Autodesk Inventor part; units mm, degrees
ref_plane "YZ Plane" through (0, 0, 0) normal (1, 0, 0) x (0, 1, 0)
ref_plane "XZ Plane" through (0, 0, 0) normal (0, 1, 0) x (-1, 0, 0)
ref_plane "XY Plane" through (0, 0, 0) normal (0, 0, 1) x (1, 0, 0)
sketch "スケッチ1" plane through (0, 0, 0) normal (0, 1, 0) x (-1, 0, 0)
  circle A0 centre (0, 0) radius 178.1675
  circle A1 centre (0, 0) radius 157.8276
  line L0 (168.1877, 0) -> (166.7488, -21.9529)
  line L1 (168.1877, 0) -> (130.1721, 2.4917) construction
  line L2 (249.4344, 0) -> (-249.4344, 0)
  line L3 (166.7488, -21.9529) -> (156.7702, -21.2989)
  line L4 (156.7702, -21.2989) -> (158.2091, 0.654) construction
  line L5 (158.2091, 0.654) -> (168.1877, 0)
  line L6 (157.4896, -10.3224) -> (0, 0)
  line L7 (166.7488, -21.9529) -> (162.4568, -43.5302)
  line L8 (162.4568, -43.5302) -> (152.649, -41.5793) construction
  line L9 (152.649, -41.5793) -> (156.9409, -20.002) construction
  line L10 (156.9409, -20.002) -> (166.7488, -21.9529) construction
  line L11 (162.4568, -43.5302) -> (155.3851, -64.3626)
  line L12 (155.3851, -64.3626) -> (145.9158, -61.1482) construction
  line L13 (145.9158, -61.1482) -> (152.9875, -40.3158) construction
  line L14 (152.9875, -40.3158) -> (162.4568, -43.5302) construction
  line L15 (155.3851, -64.3626) -> (145.6548, -84.0938)
  line L16 (145.6548, -84.0938) -> (136.6861, -79.6709) construction
  line L17 (136.6861, -79.6709) -> (146.4164, -59.9397) construction
  line L18 (146.4164, -59.9397) -> (155.3851, -64.3626) construction
  line L19 (0, 0) -> (111.6009, -111.6009)
  line L20 (145.6548, -84.0938) -> (137.3401, -78.5381) construction
  line L21 (137.3401, -78.5381) -> (125.1176, -96.8305) construction
  line L22 (125.1176, -96.8305) -> (133.4323, -102.3862) construction
  line L23 (133.4323, -102.3862) -> (145.6548, -84.0938)
  line L24 (133.4323, -102.3862) -> (125.9139, -95.7927) construction
  line L25 (125.9139, -95.7927) -> (111.4082, -112.3332) construction
  line L26 (111.4082, -112.3332) -> (118.9266, -118.9266)
  line L27 (118.9266, -118.9266) -> (133.4323, -102.3862)
  line L28 (111.6009, -111.6009) -> (118.9266, -118.9266)
  line L29 (166.7488, -21.9529) -> (176.7274, -22.6069) construction
  line L30 (118.9266, -118.9266) -> (125.9834, -125.9834)
  point P0 (154.795, -30.7906)
  point P1 (149.4517, -50.732)
  point P2 (141.5512, -69.8053)
  point P3 (131.2288, -87.6843)
  point P4 (118.661, -104.0629)
  point P5 (157.8276, 0)
  point P6 (178.1675, 0)
  dimension "d0" = 22
  dimension "d1" = 10
  dimension "d2" = 45
  dimension "d4" = 315.6551
extrude "押し出し1" add sketch "スケッチ1" along normal blind 2.5 contours L30 L27 L23 L15 L11 L7 L0 L2 A0 | L28 A1 L2 L0 L7 L11 L15 L23 L27
sketch "スケッチ2" plane through (0, 2.5, 0) normal (0, 1, 0) x (1, 0, 0)
  circle A0 centre (0, 0) radius 309.8276
  line L0 (-168.1877, 0) -> (-166.7488, 21.9529)
  line L1 (-166.7488, 21.9529) -> (-162.4568, 43.5302)
  line L2 (-162.4568, 43.5302) -> (-155.3851, 64.3626)
  line L3 (-155.3851, 64.3626) -> (-145.6548, 84.0938)
  line L4 (-133.4323, 102.3862) -> (-145.6548, 84.0938)
  line L5 (-118.9266, 118.9266) -> (-133.4323, 102.3862)
  line L6 (-167.4682, 10.9764) -> (-166.0294, 32.9293)
  line L7 (-166.0294, 32.9293) -> (-275.7938, 40.1237)
  line L8 (-275.7938, 40.1237) -> (-277.2327, 18.1708)
  line L9 (-277.2327, 18.1708) -> (-167.4682, 10.9764)
  line L10 (-164.6028, 32.7415) -> (-160.3108, 54.3188)
  line L11 (-160.3108, 54.3188) -> (-268.1972, 75.7787)
  line L12 (-268.1972, 75.7787) -> (-272.4892, 54.2015)
  line L13 (-272.4892, 54.2015) -> (-164.6028, 32.7415)
  circle A1 centre (-166.7488, 21.9529) radius 11
  circle A2 centre (-162.4568, 43.5302) radius 11
  line L14 (-158.921, 53.9464) -> (-151.8493, 74.7789)
  line L15 (-151.8493, 74.7789) -> (-256.0116, 110.1372)
  line L16 (-256.0116, 110.1372) -> (-263.0833, 89.3047)
  line L17 (-263.0833, 89.3047) -> (-158.921, 53.9464)
  circle A3 centre (-155.3851, 64.3626) radius 11
  arc A4 (-275.7591, 62.4834) -> (-281.3553, 41.7349) centre (-166.7488, 21.9529) ccw
  line L18 (-178.1663, 0.654) -> (-158.2091, -0.654)
  line L19 (-158.2091, -0.654) -> (-156.7702, 21.2989)
  line L20 (-156.7702, 21.2989) -> (-176.7274, 22.6069)
  line L21 (-176.7274, 22.6069) -> (-178.1663, 0.654)
  line L22 (-177.4468, 11.6305) -> (-275.7938, 40.1237)
  line L23 (-176.7274, 22.6069) -> (-176.008, 33.5834)
  line L24 (-176.008, 33.5834) -> (-275.7591, 62.4834)
  line L25 (-275.7938, 40.1237) -> (-281.3553, 41.7349)
  circle A5 centre (0, 0) radius 137.8276
  line L26 (0, 0) -> (-219.0812, 219.0812)
  line L27 (-111.6009, 111.6009) -> (-125.9834, 125.9834)
  line L28 (-433.7586, 0) -> (433.7586, 0)
  circle A6 centre (0, 0) radius 279.8276 construction
  arc A7 (-111.6009, 111.6009) -> (-157.8276, 0) centre (0, 0) ccw
  point P0 (-158.1662, 0)
  point P1 (-137.8276, 0)
  point P2 (-97.4588, 97.4588)
  point P3 (-309.8276, 0)
  dimension "d7" = 22
  dimension "d10" = 20
  dimension "d11" = 100
  dimension "d12" = 30
  dimension "d14" = 20
  dimension "d17" = 122
extrude "押し出し2" add sketch "スケッチ2" against normal blind 2.5 contours L26 L5 L4 L3 A3 L15 L16 L17 A2 L11 L12 L24 A4 L25 L8 L9 L21 L18 L28 A0 | L18 L21 L9 L0 | L0 A1 L19 L28 | A5 L28 A7 A1 A2 A3 L26 | L26 A7 A3 L3 L4 L5 | A1 L21 L20 L0 | L9 L21 A1 | L0 L20 L19 A1 | L19 A7 L28 | L6 A1 L1 | L20 L23 A1 L6 | L1 A1 A7 L19 L20 | L22 L7 L23 A1 L21 | L9 L8 L22 | A1 L23 L21 | A1 A7 L19 | A7 A3 L2 L3 | A3 A7 | A2 L10 L1 | A1 L7 L24 L13 | A2 A7 A1 | L13 L24 L12 L11 A2 | L1 L2 A2 A7 | A1 L23 L7 | L25 A4 L24 L12 L13 L7 | A7 A1 | A7 A2 A3 | L3 L14 A3 | L10 A2 L2 | L13 L12 L24 | A7 A2 | A3 L14 L2 | L17 L16 L15 A3
sketch "スケッチ3" plane through (0, 2.5, 0) normal (0, 1, 0) x (1, 0, 0)
  circle A0 centre (0, 0) radius 279.8276
  arc A1 (-97.4588, 97.4588) -> (-137.8276, 0) centre (0, 0) ccw
  line L0 (-97.4588, 97.4588) -> (-219.0812, 219.0812)
  line L1 (-309.8276, 0) -> (-137.8276, 0)
  arc A2 (-219.0812, 219.0812) -> (-309.8276, 0) centre (0, 0) ccw
  point P0 (-279.8276, 0)
  point P1 (-197.868, 197.868)
  dimension "d21" = 30
extrude "押し出し3" cut sketch "スケッチ3" against normal through all contours L0 A1 L1 A0 picked at (-201.5408, 115.5258)
sketch "スケッチ4" plane through (0, 2.5, 0) normal (0, 1, 0) x (1, 0, 0)
  line L0 (-279.8276, 0) -> (-309.8276, 0)
  line L1 (-286.8276, 0) -> (-309.8276, 0)
  line L2 (-309.8276, 0) -> (-309.8276, 40)
  line L3 (-309.8276, 40) -> (-286.8276, 40)
  line L4 (-286.8276, 40) -> (-286.8276, 0)
  line L5 (0, 0) -> (-232.1993, 96.1801) construction
  line L6 (-371.7931, 0) -> (61.9655, 0)
  line L7 (-197.868, 197.868) -> (-219.0812, 219.0812)
  line L8 (-202.8177, 202.8177) -> (-219.0812, 219.0812)
  line L9 (-219.0812, 219.0812) -> (-247.3654, 190.7969)
  line L10 (-247.3654, 190.7969) -> (-231.102, 174.5334)
  line L11 (-231.102, 174.5334) -> (-202.8177, 202.8177)
  dimension "d22" = 23
  dimension "d23" = 40
  dimension "d26" = 22.5
extrude "押し出し4" cut sketch "スケッチ4" against normal through all
properties part number "front_upper" material "木材 (カエデ材)"
Model file for the job. Use its own axes, mm. A direction names the side the tool comes from. Give positions to 0.01 mm unless a question says otherwise; leave off trailing zeros. Order: outer loops, then holes, each group sorted by start corner. A loop starts at its lowest first (then second) coordinate and runs counter-clockwise, first axis right, second up. Notation, with made-up numbers: (-3.5, 25) - (8.5, 25) arc R34 ccw to (8.5, 58) - close; hole circle Ø5 at (77.5, 78.5). An arc over 180 degrees is marked (long way). Return JSON: item names as keys, results as strings.
1) Cut at B-B, the plane x = -236.5. Give the cut face in (y, z).
Geometry says:
{"outline": "(0, -179.93) - (2.5, -179.93) - (2.5, -149.57) - (0, -149.57) - close"}
2) Probe line 1 (Z direction, x = -281, y = 0.1); line 2 (Z direction, x = -238.5, y = 0.8); line 3 (X direction, y = 0.45, z = -175). List the from-to ranges inside material, lowest first. Write a range as from..to.
Geometry says:
{"line 1": "-130.51..0", "line 2": "-181.93..-146.36", "line 3": "-255.67..-231.57, -230.64..-218.35"}
3) Cut at A-A, the plane y = 1. Give the cut face in (x, z).
Geometry says:
{"outline": "(-307.23, -40) arc R309.83 ccw to (-245.53, -188.96) - (-231.1, -174.53) - (-202.82, -202.82) - (-197.87, -197.87) arc R279.83 cw to (-279.83, 0) - (-286.83, 0) - (-286.83, -40) - close"}
4) Cut at C-C, the plane z = -58. Give the cut face in (x, y).
Geometry says:
{"outline": "(-304.35, 0) - (-273.75, 0) - (-273.75, 2.5) - (-304.35, 2.5) - close"}
5) 3-axis set-ups, long thin cutter, end or side, ignore diameter. For faces 1 (the flat face through (-269, 2.5, -109)), 2 (the flat face through (-238.42, 1.27, -181.85)): which of +Z, -Z, +X, -X, +Y, -Y reach the whole face in a straight line?
Geometry says:
{"face 1": "+Z, -Z, +X, -X, +Y", "face 2": "-Z, +Y, -Y"}
6) Pull direction X, two halves, no side cores. Call faces 3 (the cylindrical face through (-285.804, 1.268, -119.62)), 4 (the flat face through (-217.158, 1.268, -188.478)), 5 (the cylindrical face through (-257.934, 1.268, -108.505)), 6 (the flat face through (-269, 0, -109)): pulls with the +X half, pulls with the -X half, needs draft (parallel to the pull), parting line crosses it, or undercut.
Geometry says:
{"face 3": "pulls with the -X half", "face 4": "undercut", "face 5": "pulls with the +X half", "face 6": "needs draft"}
